Here's how the part is built. I have some questions about the finished solid (model axes, mm). A direction names the side the tool comes from. Coordinates: 2 decimals unless noted, no trailing zeros. Write each loop counter-clockwise with the first axis right and the second up, starting at its lowest first coordinate (ties: lowest second). Pieces come first, ordered by that corner, then holes. Notation, with made-up numbers: M -36,45 L 9,45 A12 cw 9,66 Z; hole C 16,50.5 d9. An arc over 180 degrees is marked long. Use a Markdown table: item, result.
```python
from build123d import *

# Parameters (mm, degrees)
F1_DEPTH = 10
F2_R     = 3.5
F4_DEPTH = 1
F3_R     = 3.5
F6_DEPTH = 1


# Not quite as in the source:
# - a fillet or chamfer that OpenCascade refuses, or shapes differently, is made with other operations: its cross-section is extruded or revolved along the edge and cut away or added


with BuildPart() as f1:
    # F0 (on Top) → F1 (new body)
    with BuildSketch(Plane.XY):
        with BuildLine():
            Line((-7.0290866446, 4), (-2.3094010768, 4))
            Line((-2.3094010768, 4), (2.3094010768, 4))
            Line((2.3094010768, 4), (7.0290866446, 4))
            ThreePointArc((7.0290866446, 4), (0, 8.087524903), (-7.0290866446, 4))
        make_face()
        with BuildLine():
            Line((-4.6188021535, 0), (-2.3094010768, 4))
            Line((-2.3094010768, 4), (-7.0290866446, 4))
            ThreePointArc((-7.0290866446, 4), (-8.087524903, 0), (-7.0290866446, -4))
            Line((-7.0290866446, -4), (-2.3094010768, -4))
            Line((-2.3094010768, -4), (-4.6188021535, 0))
        make_face()
        with BuildLine():
            Line((7.0290866446, 4), (2.3094010768, 4))
            Line((2.3094010768, 4), (4.6188021535, 0))
            Line((4.6188021535, 0), (2.3094010768, -4))
            Line((2.3094010768, -4), (7.0290866446, -4))
            ThreePointArc((7.0290866446, -4), (7.8184388576, -2.068833702), (8.087524903, 0))
            ThreePointArc((8.087524903, 0), (7.8184388576, 2.068833702), (7.0290866446, 4))
        make_face()
        with BuildLine():
            ThreePointArc((-7.0290866446, -4), (-8.087524903, 0), (-7.0290866446, 4))
            Line((-7.0290866446, 4), (-21, 4))
            ThreePointArc((-21, 4), (-23.8284271247, 2.8284271247), (-25, 0))
            ThreePointArc((-25, 0), (-23.8284271247, -2.8284271247), (-21, -4))
            Line((-21, -4), (-7.0290866446, -4))
        make_face()
        with BuildLine():
            Line((21, 4), (7.0290866446, 4))
            ThreePointArc((7.0290866446, 4), (7.8184388576, 2.068833702), (8.087524903, 0))
            ThreePointArc((8.087524903, 0), (7.8184388576, -2.068833702), (7.0290866446, -4))
            Line((7.0290866446, -4), (21, -4))
            ThreePointArc((21, -4), (23.8284271247, -2.8284271247), (25, 0))
            ThreePointArc((25, 0), (23.8284271247, 2.8284271247), (21, 4))
        make_face()
        with BuildLine():
            Line((2.3094010768, -4), (-2.3094010768, -4))
            Line((-2.3094010768, -4), (-7.0290866446, -4))
            ThreePointArc((-7.0290866446, -4), (0, -8.087524903), (7.0290866446, -4))
            Line((7.0290866446, -4), (2.3094010768, -4))
        make_face()
    extrude(amount=F1_DEPTH)

    # F2 (on face) → F4 (cut)
    with BuildSketch(Plane.XZ.offset(4)):
        with Locations((-14.1732281117, 5)):
            Circle(F2_R)
        with Locations((14.1732281117, 5)):
            Circle(F2_R)
    extrude(amount=-F4_DEPTH, mode=Mode.SUBTRACT)

    # F5: fillet of radius 5 on 2 edges, made by hand

    # F5_s1 → F5_t2 (revolve)
    with BuildSketch(Plane.XY.offset(5)):
        with BuildLine():
            ThreePointArc((-10.6732281117, -4), (-12.0920892816, -3.2565835097), (-13.6732281117, -3))
            Line((-13.6732281117, -3), (-10.6732281117, -3))
            Line((-10.6732281117, -3), (-10.6732281117, -4))
        make_face()
    revolve(axis=Axis((-14.1732281117, -3, 5), (0, -1, 0)))

    # F5_s3 → F5_t4 (revolve)
    with BuildSketch(Plane.XY.offset(5)):
        with BuildLine():
            ThreePointArc((17.6732281117, -4), (16.2543669417, -3.2565835097), (14.6732281117, -3))
            Line((14.6732281117, -3), (17.6732281117, -3))
            Line((17.6732281117, -3), (17.6732281117, -4))
        make_face()
    revolve(axis=Axis((14.1732281117, -3, 5), (0, -1, 0)))

    # F3 (on face) → F6 (cut)
    with BuildSketch(Plane(origin=(0, 4, 0), x_dir=(-1, 0, 0), z_dir=(0, 1, 0))):
        with Locations((13.4998997673, 5.0000185147)):
            Circle(F3_R)
        with Locations((-13.4998997673, 5.0000185147)):
            Circle(F3_R)
    extrude(amount=-F6_DEPTH, mode=Mode.SUBTRACT)

    # F7: fillet of radius 5 on 2 edges, made by hand

    # F7_s1 → F7_t2 (revolve)
    with BuildSketch(Plane.XY.offset(5.0000185147)):
        with BuildLine():
            ThreePointArc((9.9998997673, 4), (11.4187609373, 3.2565835097), (12.9998997673, 3))
            Line((12.9998997673, 3), (9.9998997673, 3))
            Line((9.9998997673, 3), (9.9998997673, 4))
        make_face()
    revolve(axis=Axis((13.4998997673, 3, 5.0000185147), (0, 1, 0)))

    # F7_s3 → F7_t4 (revolve)
    with BuildSketch(Plane.XY.offset(5.0000185147)):
        with BuildLine():
            ThreePointArc((-16.9998997673, 4), (-15.5810385974, 3.2565835097), (-13.9998997673, 3))
            Line((-13.9998997673, 3), (-16.9998997673, 3))
            Line((-16.9998997673, 3), (-16.9998997673, 4))
        make_face()
    revolve(axis=Axis((-13.4998997673, 3, 5.0000185147), (0, 1, 0)))


solid = f1.part
```
1. Which directions (+Z, -Z, +X, -X, +Y, -Y) give clear straight access to the entire face, cutting with the end or side of a thin tool? Please do faces 1 (the face through (-14, -3, 5)), 2 (the face through (12, -4, 2)), 3 (the face through (-12.6, -4, 1.6)).
Answers follow:
| item | result |
|---|---|
| face 1 | -Y |
| face 2 | +Z, -Z, +X, -Y |
| face 3 | +Z, -Z, -X, -Y |
2. Suppose I cut it at B-B on y = 1. Write out the boundary of the cut face in (x, z), and give its area (3 significant figures).
Answers follow:
| item | result |
|---|---|
| outline | M -24.87,0 L -4.04,0 L -4.04,10 L -24.87,10 Z; M 4.04,0 L 24.87,0 L 24.87,10 L 4.04,10 Z |
| area | 417 mm2 |
3. Suppose I cut it at D-D on y = 5.5. Write out the boundary of the cut face in (x, z).
Answers follow:
| item | result |
|---|---|
| outline | M -5.93,0 L 5.93,0 L 5.93,10 L -5.93,10 Z |
4. Suppose I cut it at A-A on x = 3.5. Write out the boundary of the cut face in (y, z).
Answers follow:
| item | result |
|---|---|
| outline | M -7.29,0 L -1.94,0 L -1.94,10 L -7.29,10 Z; M 1.94,0 L 7.29,0 L 7.29,10 L 1.94,10 Z |
5. We'd pull the mould along Y, two halves only. Please class faces 4 (the face through (0, 4, 5)), 5 (the face through (17.2, 4, 4.9)), 6 (the face through (-3.48, 1.97, 4.93)), 7 (the face through (5, 0, 10)): +Y half, -Y half, draft (parallel to the pull), parting line (faces both ways), or undercut.
Answers follow:
| item | result |
|---|---|
| face 4 | undercut |
| face 5 | +Y half |
| face 6 | undercut |
| face 7 | draft |
6. Will these pins go through, and if not, where does the flat tip stop? pin 1 Ø3 at (x, z) = (-12, 4.5) entering from -Y; pin 2 Ø4 at (y, z) = (5, 7) entering from -X; pin 3 Ø1 at (y, z) = (1, 6) entering from +X.
Answers follow:
| item | result |
|---|---|
| pin 1 | stops at y = -4 |
| pin 2 | stops at x = -23.65 |
| pin 3 | stops at x = 24.97 |
7. I need wall thicknesses on probe 1 along Y at (x, z) = (8, 6.75); probe 2 along X at (y, z) = (-3.5, 6); probe 3 along X at (y, z) = (-1.5, 4.5). Which ranges of each line are inside material? Lowest first, please.
Answers follow:
| item | result |
|---|---|
| probe 1 | y = -4 to 4 |
| probe 2 | x = -22.94 to -16.66, -11.69 to -2.6, 2.6 to 11.69, 16.66 to 22.94 |
| probe 3 | x = -24.71 to -3.75, 3.75 to 24.71 |
8. Suppose I cut it at C-C on x = 20. Write out the boundary of the cut face in (y, z).
Answers follow:
| item | result |
|---|---|
| outline | M -4,0 L 4,0 L 4,10 L -4,10 Z |
